from build123d import *

# Parameters (mm, degrees)
ESQUISSE1_W        = 680
ESQUISSE1_H        = 90
ESQUISSE1_R        = 2.75
ESQUISSE1_R_2      = 14
ESQUISSE1_R_3      = 4
BOSS_EXTRU_1_DEPTH = 8
ESQUISSE2_W        = 8
ESQUISSE2_H        = 90
BOSS_EXTRU_2_DEPTH = 20
ESQUISSE3_W        = 8
ESQUISSE3_H        = 90
BOSS_EXTRU_3_DEPTH = 20


with BuildPart() as part:
    # Esquisse1 → Boss.-Extru.1 (new body)
    with BuildSketch(Plane.XY):
        with Locations((340, 45)):
            Rectangle(ESQUISSE1_W, ESQUISSE1_H)
        with Locations((317, 48.92)):
            Circle(ESQUISSE1_R, mode=Mode.SUBTRACT)
        with Locations((363, 48.92)):
            Circle(ESQUISSE1_R, mode=Mode.SUBTRACT)
        with Locations((363, 30.92)):
            Circle(ESQUISSE1_R, mode=Mode.SUBTRACT)
        with Locations((317, 30.92)):
            Circle(ESQUISSE1_R, mode=Mode.SUBTRACT)
        with Locations((340, 48.92)):
            Circle(ESQUISSE1_R_2, mode=Mode.SUBTRACT)
        with Locations((35.3, 75)):
            Circle(ESQUISSE1_R_3, mode=Mode.SUBTRACT)
        with Locations((35.3, 45)):
            Circle(ESQUISSE1_R_3, mode=Mode.SUBTRACT)
        with Locations(Location((644.7, 45, 0), (0, 0, 180))):
            Circle(ESQUISSE1_R_3, mode=Mode.SUBTRACT)
        with Locations(Location((644.7, 75, 0), (0, 0, 180))):
            Circle(ESQUISSE1_R_3, mode=Mode.SUBTRACT)
        with Locations((155.3, 75)):
            Circle(ESQUISSE1_R_3, mode=Mode.SUBTRACT)
        with Locations((155.3, 45)):
            Circle(ESQUISSE1_R_3, mode=Mode.SUBTRACT)
        with Locations((275.3, 75)):
            Circle(ESQUISSE1_R_3, mode=Mode.SUBTRACT)
        with Locations((275.3, 45)):
            Circle(ESQUISSE1_R_3, mode=Mode.SUBTRACT)
        with Locations(Location((404.7, 45, 0), (0, 0, 180))):
            Circle(ESQUISSE1_R_3, mode=Mode.SUBTRACT)
        with Locations(Location((404.7, 75, 0), (0, 0, 180))):
            Circle(ESQUISSE1_R_3, mode=Mode.SUBTRACT)
        with Locations(Location((524.7, 45, 0), (0, 0, 180))):
            Circle(ESQUISSE1_R_3, mode=Mode.SUBTRACT)
        with Locations(Location((524.7, 75, 0), (0, 0, 180))):
            Circle(ESQUISSE1_R_3, mode=Mode.SUBTRACT)
    extrude(amount=BOSS_EXTRU_1_DEPTH)

    # Esquisse2 → Boss.-Extru.2 (add)
    with BuildSketch(Plane.ZY):
        with Locations((4, 45)):
            Rectangle(ESQUISSE2_W, ESQUISSE2_H)
    extrude(amount=BOSS_EXTRU_2_DEPTH)

    # Esquisse3 → Boss.-Extru.3 (add)
    with BuildSketch(Plane(origin=(680, 0, 0), x_dir=(0, 0, -1), z_dir=(1, 0, 0))):
        with Locations((-4, 45)):
            Rectangle(ESQUISSE3_W, ESQUISSE3_H)
    extrude(amount=BOSS_EXTRU_3_DEPTH)


solid = part.part
Can you work these out from the model? Positions are in its coordinate system, mm. Give positions to 0.01 mm unless a question says otherwise; leave off trailing zeros. Write each loop counter-clockwise with the first axis right and the second up, starting at its lowest first coordinate (ties: lowest second). Pieces come first, ordered by that corner, then holes. Notation, with made-up numbers: M 26.25,-13.5 L 69.25,-13.5 A20 cw 69.25,2.5 Z; hole C 39.5,62.25 d4. An arc over 180 degrees is marked long. Answer in a Markdown table with one row per item. Add a question column.
Item 1: For pin 1 Ø7 at (x, y) = (404.7, 45) entering from -Z; pin 2 Ø9 at (x, y) = (275.3, 45) entering from +Z, each with a flat end and sliding along its axis, tell me the tip position at first contact or that it passes through.
Item 2: We'd pull the mould along Y, two halves only. Please class faces 1 (the cylindrical face through (352.932, 43.558, 3.944)), 2 (the flat face through (335, 34, 8)): released by +Y, released by -Y, zero draft, split by the parting line, or undercut.
Item 3: Imagine slicing it at B-B, the plane x = 340. Write out the boundary of the cut face in (y, z).
Item 4: Please list where these lines run through material, in increasing order: L1, parallel to Y at x = 317, z = 3; L2, parallel to Y at x = 404.7, z = 2; L3, parallel to X at y = 60, z = 4.5.
Item 5: Imagine slicing it at A-A, the plane z = 2.25. State how many separate pieces and enclosed holes the cut face has, plus the area to 3 significant figures.
Evaluation:
| question | item | result |
|---|---|---|
| 1 | pin 1 | passes through |
| 1 | pin 2 | stops at z = 8 |
| 2 | face 1 | undercut |
| 2 | face 2 | zero draft |
| 3 | outline | M 0,0 L 34.92,0 L 34.92,8 L 0,8 Z; M 62.92,0 L 90,0 L 90,8 L 62.92,8 Z |
| 4 | L1 | y = 0 to 28.17, 33.67 to 46.17, 51.67 to 90 |
| 4 | L2 | y = 0 to 41, 49 to 71, 79 to 90 |
| 4 | L3 | x = -20 to 331.44, 348.56 to 700 |
| 5 | separate pieces | 1 |
| 5 | enclosed holes | 17 |
| 5 | area | 63,500 mm² |
